Read the model definition and answer for the solid it produces. Units are mm, in the model's axes. A direction names the side the tool comes from. Coordinates: 2 decimals unless noted, no trailing zeros. Write each loop counter-clockwise with the first axis right and the second up, starting at its lowest first coordinate (ties: lowest second). Pieces come first, ordered by that corner, then holes.
1) The part is cut by section D-D (z = -110.5). Determine the outline of the cut face in (x, y).
2) The part is cut by section B-B (x = -26). Determine the outline of the cut face in (y, z).
3) Each of these flat-tipped pins is pushed along its axis until it touches: pin 1 Ø3 at (y, z) = (-1, -92) entering from -X; pin 2 Ø1.5 at (x, y) = (-62, 4.5) entering from +Z; pin 3 Ø3 at (x, y) = (-57.5, 0) entering from +Z. Where does it stop, or does it pass through?
4) Find the intervals of material crossed by line 1 (Z direction, x = -76.5, y = 3) (3 decimals); line 2 (Z direction, x = -35, y = 2.75); line 3 (Z direction, x = -32, y = 3.25), in increasing order.
5) The part is cut by section C-C (x = -87). Determine the outline of the cut face in (y, z) (3 decimals), then the cut area to 3 significant figures.
6) Which of the six approach directions +Z, -Z, +X, -X, +Y, -Y give full straight-line access (tool end or side, diameter ignored) to faces 1 (the face through (-83, 0, -3.175)), 2 (the face through (-83, 0, 0)), 3 (the face through (-44.58, -0.09, -42.72))?
7) Determine the mould class of faces 4 (the face through (-57.99, 0.1, -16.37)), 5 (the face through (-19.67, -0.09, -81.26)), 6 (the face through (-66.03, -0.089, -0.874)) for opening direction Z: +Z half, -Z half, draft (parallel to the pull), parting line (faces both ways), or undercut.
from build123d import *

# Parameters (mm, degrees)
ESBO_O2_W               = 193.5
ESBO_O2_H               = 12.7
FLANGE_BASE1_DEPTH      = 3.175
DOBRA_START             = -6.35
DOBRA_ESBO_ADA1_DEPTH   = 12.7
DOBRA_ESBO_ADA1_2_DEPTH = 12.7
DOBRA_ESBO_ADA2_DEPTH   = 12.7
DOBRA_ESBO_ADA2_2_DEPTH = 12.7
ESBO_O10_R              = 2.75
CORTE_EXTRUS_O2_DEPTH   = 10
ESBO_O11_R              = 2.75
CORTE_EXTRUS_O3_DEPTH   = 10
ESBO_O12_R              = 1.65
ESBO_O12_R_2            = 2.250000002
CORTE_EXTRUS_O4_DEPTH   = 10


# Read off the part's stored shape, not the designer's step: Dobra esboçada1, Dobra esboçada2
# Sheet-metal steps are written as plain solids
with BuildPart() as part:
    # Esboço2 → Flange-base1 (new body)
    with BuildSketch(Plane.XY):
        Rectangle(ESBO_O2_W, ESBO_O2_H)
    extrude(amount=-FLANGE_BASE1_DEPTH)

    # Dobra esboçada1 outline → Dobra esboçada1 (cut)
    with BuildSketch(Plane(origin=(0, 0, 0), x_dir=(1, 0, 0), z_dir=(0, 1, 0)).offset(DOBRA_START)):
        with BuildLine():
            Line((96.75, 3.175), (-63.744109855, 3.175))
            ThreePointArc((-63.744109855, 3.175), (-66.070007409, 0.850686918), (-69.246257163, 0))
            Line((-69.246257163, 0), (96.75, 0))
            Line((96.75, 0), (96.75, 3.175))
        make_face()
    extrude(amount=DOBRA_ESBO_ADA1_DEPTH, mode=Mode.SUBTRACT)

    # Dobra esbo_ada1 2 outline → Dobra esbo_ada1 2 (add)
    with BuildSketch(Plane(origin=(0, 0, 0), x_dir=(1, 0, 0), z_dir=(0, 1, 0)).offset(DOBRA_START)):
        with BuildLine():
            Line((16.759205697, 142.610831402), (14.00957504, 144.198331402))
            Line((14.00957504, 144.198331402), (-66.492296379, 4.765))
            ThreePointArc((-66.492296379, 4.765), (-67.656257163, 3.601039216), (-69.246257163, 3.175))
            Line((-69.246257163, 3.175), (-63.744109855, 3.175))
            ThreePointArc((-63.744109855, 3.175), (-63.743387647, 3.176249918), (-63.742665722, 3.1775))
            Line((-63.742665722, 3.1775), (16.759205697, 142.610831402))
        make_face()
    extrude(amount=DOBRA_ESBO_ADA1_2_DEPTH)

    # Dobra esboçada2 outline → Dobra esboçada2 (cut)
    with BuildSketch(Plane(origin=(0, 0, 0), x_dir=(1, 0, 0), z_dir=(0, 1, 0)).offset(DOBRA_START)):
        with BuildLine():
            Line((14.00957504, 144.198331402), (-20.519351306, 84.39247664))
            ThreePointArc((-20.519351306, 84.39247664), (-19.669385908, 81.21603373), (-20.520794303, 78.039977295))
            Line((-20.520794303, 78.039977295), (16.759205697, 142.610831402))
            Line((16.759205697, 142.610831402), (14.00957504, 144.198331402))
        make_face()
    extrude(amount=DOBRA_ESBO_ADA2_DEPTH, mode=Mode.SUBTRACT)

    # Dobra esbo_ada2 2 outline → Dobra esbo_ada2 2 (add)
    with BuildSketch(Plane(origin=(0, 0, 0), x_dir=(1, 0, 0), z_dir=(0, 1, 0)).offset(DOBRA_START)):
        with BuildLine():
            Line((-58.054167797, 143.054687167), (-23.27042496, 82.807477295))
            ThreePointArc((-23.27042496, 82.807477295), (-22.844385744, 81.217477295), (-23.27042496, 79.627477295))
            Line((-23.27042496, 79.627477295), (-20.519351306, 84.39247664))
            ThreePointArc((-20.519351306, 84.39247664), (-20.520072663, 84.393727049), (-20.520794303, 84.394977295))
            Line((-20.520794303, 84.394977295), (-55.30453714, 144.642187167))
            Line((-55.30453714, 144.642187167), (-58.054167797, 143.054687167))
        make_face()
    extrude(amount=DOBRA_ESBO_ADA2_2_DEPTH)

    # Esboço10 → Corte-extrusão2 (cut)
    with BuildSketch(Plane(origin=(18.403870761, 0, -10.625479738), x_dir=(0.5000000000000041, 0, 0.8660254037844364), z_dir=(-0.8660254037844363, 0, 0.500000000000004))):
        with Locations((-144.864192108, 0)):
            Circle(ESBO_O10_R)
    extrude(amount=-CORTE_EXTRUS_O2_DEPTH, mode=Mode.SUBTRACT)

    # Esboço11 → Corte-extrusão3 (cut)
    with BuildSketch(Plane(origin=(0, 0, -3.175), x_dir=(-1, 0, 0), z_dir=(0, 0, -1))):
        with Locations((77.77220064, 0)):
            Circle(ESBO_O11_R)
    extrude(amount=-CORTE_EXTRUS_O3_DEPTH, mode=Mode.SUBTRACT)

    # Esboço12 → Corte-extrusão4 (cut)
    with BuildSketch(Plane(origin=(-51.932527808, 0, -29.98325891), x_dir=(-0.49999999999999806, 0, 0.8660254037844398), z_dir=(-0.8660254037844397, 0, -0.499999999999998))):
        with Locations((-27.332391374, 0.04)):
            Circle(ESBO_O12_R)
        with Locations((17.064458437, 0)):
            Circle(ESBO_O12_R_2)
        with Locations((-9.431391374, 0.04)):
            Circle(ESBO_O12_R)
    extrude(amount=-CORTE_EXTRUS_O4_DEPTH, mode=Mode.SUBTRACT)


solid = part.part
Reported:
1. outline: (-39.26, -6.35) - (-35.59, -6.35) - (-35.59, 6.35) - (-39.26, 6.35) - close
2. outline: (-6.35, -93.89) - (6.35, -93.89) - (6.35, -87.54) - (-6.35, -87.54) - close; (-6.35, -74.9) - (6.35, -74.9) - (6.35, -68.55) - (-6.35, -68.55) - close
3. pin 1: stops at x = -29.44
3. pin 2: stops at z = -4.9
3. pin 3: stops at z = -11.39
4. line 1: z = -3.175 to 0
4. line 2: z = -109.47 to -103.12, -59.31 to -52.96
4. line 3: z = -104.28 to -97.93, -64.51 to -58.16
5. outline: (-6.35, -3.175) - (6.35, -3.175) - (6.35, 0) - (-6.35, 0) - close
5. area: 40.3 mm2
6. face 1: -Z, -X, +Y, -Y
6. face 2: +Z, +X, -X, +Y, -Y
6. face 3: -X, +Y, -Y
7. face 4: undercut
7. face 5: parting line
7. face 6: +Z half
